Drawing for the job (mm, zero at the part's lowest x, y, z). Round coordinates to 2 decimals unless told otherwise and drop trailing zeros. Loops run counter-clockwise (first coordinate to the right, second up) from the corner with the lowest first, then second, coordinate; pieces in that order, holes last. Notation, with made-up numbers: M 33,84.5 L 51,84.5 A9 ccw 51,100.5 Z; hole C 86,16 d3. An arc over 180 degrees is marked long. Answer in a Markdown table with one row per item.
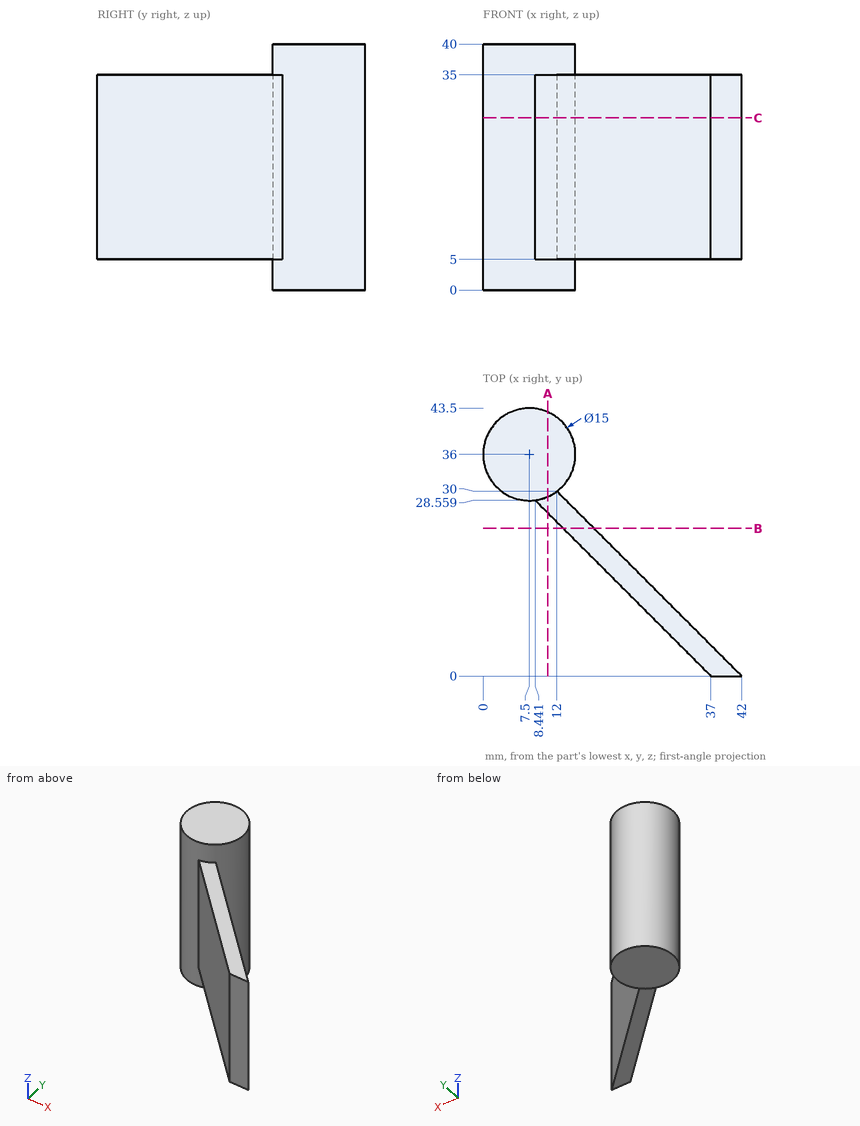
1. Wall check: probe 1 along Z at (x, y) = (24, 15); probe 2 along Y at (x, z) = (4, 24.5); probe 3 along Y at (x, z) = (9, 31). Give the ranges that are in metal, low to high.
Verdict:
| item | result |
|---|---|
| probe 1 | z = 5 to 35 |
| probe 2 | y = 29.37 to 42.63 |
| probe 3 | y = 28 to 43.35 |
2. Saw through at C-C (z = 28). Write the cut outline in (x, y).
Verdict:
| item | result |
|---|---|
| outline | M 8.44,28.56 L 37,0 L 42,0 L 12,30 A7.5 ccw long Z |
3. Saw through at A-A (x = 10.5). Write the cut outline in (y, z), and give its area (3 significant figures).
Verdict:
| item | result |
|---|---|
| outline | M 26.5,5 L 29.13,5 L 29.13,0 L 42.87,0 L 42.87,40 L 29.13,40 L 29.13,35 L 26.5,35 Z |
| area | 629 mm² |
4. Saw through at B-B (y = 24). Write the cut outline in (x, z).
Verdict:
| item | result |
|---|---|
| outline | M 13,5 L 18,5 L 18,35 L 13,35 Z |
5. Pin check, flat tips, straight feed: pin 1 (1.5 mm diameter, centred on x = 33.5, z = 9.5, fed in from +Y); pin 2 (24 mm diameter, centred on x = 27, y = 18, fed in from +Z); pin 3 (10 mm diameter, centred on x = 16, z = 10.5, fed in from +Y); pin 4 (2 mm diameter, centred on x = 18.5, y = 16.5, fed in from +Z). Stop position of each tip, or through.
Verdict:
| item | result |
|---|---|
| pin 1 | stops at y = 9.25 |
| pin 2 | stops at z = 35 |
| pin 3 | stops at y = 42.63 |
| pin 4 | passes through |
